Here's the drawing with two shaded views (mm, measured from the low corner). I have some questions. Round coordinates to 2 decimals unless told otherwise and drop trailing zeros. Order: outer loops, then holes, each group sorted by start corner. A loop starts at its lowest first (then second) coordinate and runs counter-clockwise, first axis right, second up.
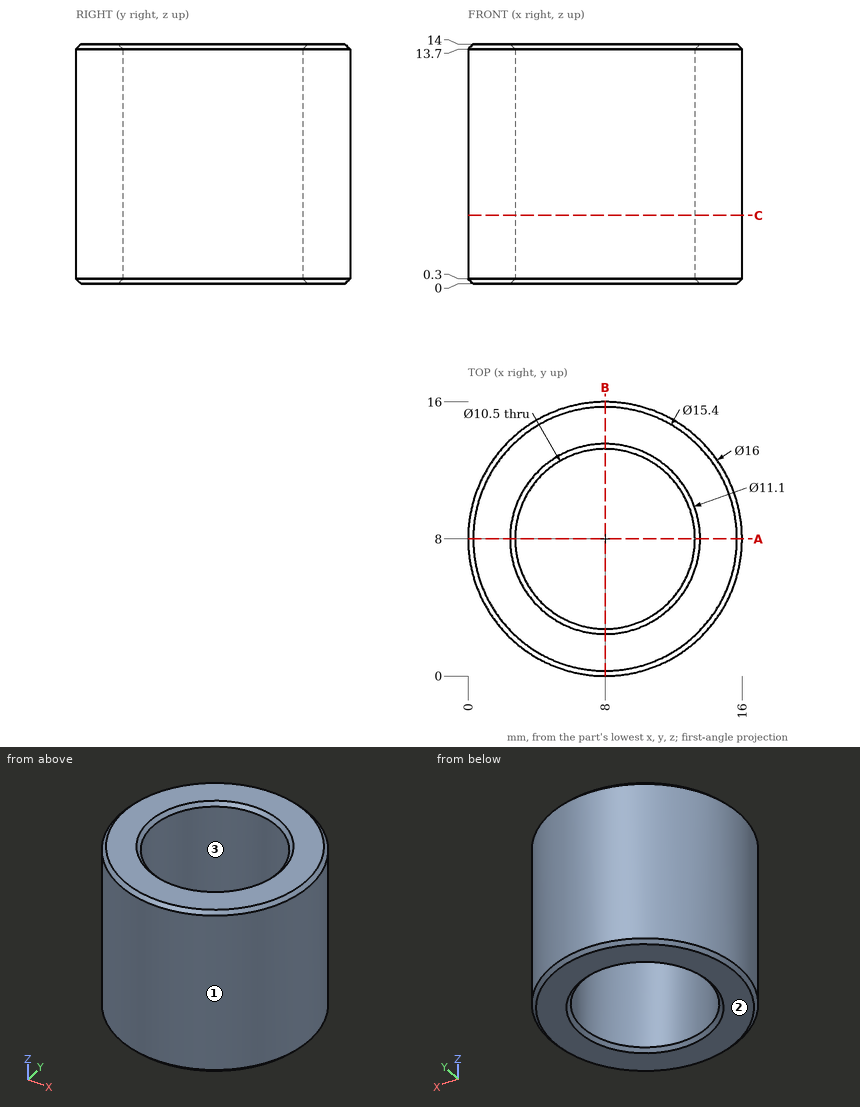
Q1. Imagine slicing it at C-C, the plane z = 4. Please give me the cut outline in (x, y), then the cut area to 3 significant figures.
Q2. Imagine slicing it at A-A, the plane y = 8. Please give me the cut outline in (x, z).
Q3. I need wall thicknesses on L1, parallel to Y at x = 8, z = 9.5; L2, parallel to Y at x = 4, z = 6.25; L3, parallel to X at y = 8.5, z = 7. Which ranges of each line are inside material? Lowest first, please.
Q4. For P1, Ø1, axis at x = 10, z = 9.5, coming from the +Y side; P2, Ø4, axis at y = 14, z = 2.5, coming from the -X side; P3, Ø4, axis at y = 13.5, z = 3.5, coming from the -X side; P4, Ø6, axis at x = 6.5, y = 9.5, coming from the -Z side, each with a flat end and sliding along its axis, tell me the tip position at first contact or that it passes through.
Q5. We'd pull the mould along X, two halves only. Please class the marked faces 1, 2 and 3: released by +X, released by -X, zero draft, split by the parting line, or undercut.
Filled in:
1. outline: circle Ø16 at (8, 8); hole circle Ø10.5 at (8, 8)
1. area: 114 mm2
2. outline: (0, 0.3) - (0.3, 0) - (2.45, 0) - (2.75, 0.3) - (2.75, 13.7) - (2.45, 14) - (0.3, 14) - (0, 13.7) - close; (13.25, 0.3) - (13.55, 0) - (15.7, 0) - (16, 0.3) - (16, 13.7) - (15.7, 14) - (13.55, 14) - (13.25, 13.7) - close
3. L1: y = 0 to 2.75, 13.25 to 16
3. L2: y = 1.07 to 4.6, 11.4 to 14.93
3. L3: x = 0.02 to 2.77, 13.23 to 15.98
4. P1: stops at y = 15.86
4. P2: stops at x = 1.07
4. P3: stops at x = 0.81
4. P4: passes through
5. face 1: split by the parting line
5. face 2: zero draft
5. face 3: undercut
